Part model, mm, in its own coordinate system. Face numbers are marked on the shaded views. A direction names the side the tool comes from. Give positions to 0.01 mm unless a question says otherwise; leave off trailing zeros. Order: outer loops, then holes, each group sorted by start corner. A loop starts at its lowest first (then second) coordinate and runs counter-clockwise, first axis right, second up. Notation, with made-up numbers: M 26,33 L 31,33 A30 cw 31,58 Z; hole C 49.25,3.25 d8. An arc over 180 degrees is marked long. Return JSON: item names as keys, results as strings.
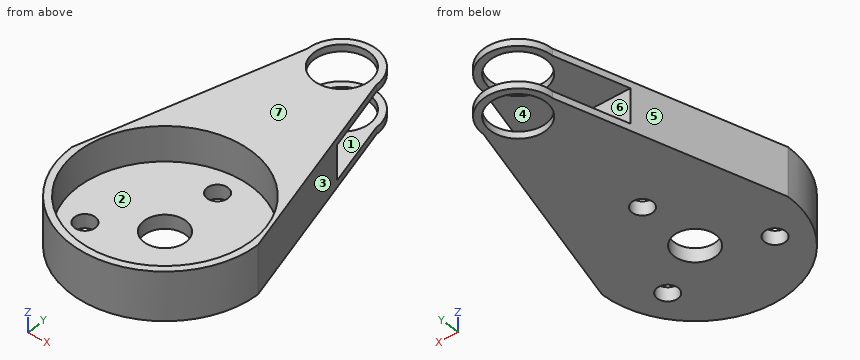
from build123d import *

# Parameters (mm, degrees)
BOSS_EXTRU_1_DEPTH      = 7
ESQUISSE2_R             = 3
ENL_V_MAT_EXTRU_1_DEPTH = 7
ESQUISSE3_R             = 1.5
ENL_V_MAT_EXTRU_2_DEPTH = 7
ESQUISSE4_R             = 4
ENL_V_MAT_EXTRU_3_DEPTH = 7
ESQUISSE5_R             = 12.5
ENL_V_MAT_EXTRU_4_DEPTH = 5
ESQUISSE6_W             = 27
ESQUISSE6_H             = 5
ENL_V_MAT_EXTRU_5_DEPTH = 20


with BuildPart() as part:
    # Esquisse1 → Boss.-Extru.1 (new body)
    with BuildSketch(Plane.XY):
        with BuildLine():
            Line((5, 0), (13.5, -30.265491901))
            ThreePointArc((13.5, -30.265491901), (0, -43.765491901), (-13.5, -30.265491901))
            Line((-13.5, -30.265491901), (-5, 0))
            ThreePointArc((-5, 0), (0, 5), (5, 0))
        make_face()
    extrude(amount=BOSS_EXTRU_1_DEPTH)

    # Esquisse2 → Enlèv. mat.-Extru.1 (cut)
    with BuildSketch(Plane.XY.offset(7)):
        with Locations((0, -30.265491901)):
            Circle(ESQUISSE2_R)
    extrude(amount=-ENL_V_MAT_EXTRU_1_DEPTH, mode=Mode.SUBTRACT)

    # Esquisse3 → Enlèv. mat.-Extru.2 (cut)
    with BuildSketch(Plane.XY.offset(7)):
        with Locations((0, -21.265491901)):
            Circle(ESQUISSE3_R)
        with Locations((-7.794228634, -34.765491901)):
            Circle(ESQUISSE3_R)
        with Locations((7.794228634, -34.765491901)):
            Circle(ESQUISSE3_R)
    extrude(amount=-ENL_V_MAT_EXTRU_2_DEPTH, mode=Mode.SUBTRACT)

    # Esquisse4 → Enlèv. mat.-Extru.3 (cut)
    with BuildSketch(Plane.XY.offset(7)):
        Circle(ESQUISSE4_R)
    extrude(amount=-ENL_V_MAT_EXTRU_3_DEPTH, mode=Mode.SUBTRACT)

    # Esquisse5 → Enlèv. mat.-Extru.4 (cut)
    with BuildSketch(Plane.XY.offset(7)):
        with Locations((0, -30.265491901)):
            Circle(ESQUISSE5_R)
    extrude(amount=-ENL_V_MAT_EXTRU_4_DEPTH, mode=Mode.SUBTRACT)

    # Esquisse6 → Enlèv. mat.-Extru.5 (cut)
    with BuildSketch(Plane(origin=(0, 10, 0), x_dir=(1, 0, 0), z_dir=(0, 1, 0))):
        with Locations((0, -3.5)):
            Rectangle(ESQUISSE6_W, ESQUISSE6_H)
    extrude(amount=-ENL_V_MAT_EXTRU_5_DEPTH, mode=Mode.SUBTRACT)


solid = part.part
Q1. Probe line 1 along Y through (x, z) = (0, 0.65); line 2 along Y through (x, z) = (0, 6.45); line 3 along Y through (x, z) = (0, 4.1). List the from-to ranges inside material, lowest first.
Established:
{"line 1": "y = -43.77 to -33.27, -27.27 to -22.77, -19.77 to -4, 4 to 5", "line 2": "y = -43.77 to -42.77, -17.77 to -4, 4 to 5", "line 3": "y = -43.77 to -42.77, -17.77 to -10"}
Q2. Band-saw the part on C-C (y = -32.5). Give the cut face in (x, z).
Established:
{"outline": "M -13.31,0 L -2,0 L -2,2 L -12.3,2 L -12.3,7 L -13.31,7 Z; M 2,0 L 13.31,0 L 13.31,7 L 12.3,7 L 12.3,2 L 2,2 Z"}
Q3. Band-saw the part on B-B (z = 3.5). Give the cut face in (x, y), then the cut area to 3 significant figures.
Established:
{"outline": "M -13.5,-30.27 A13.5 ccw 13.5,-30.27 L 7.81,-10 L -7.81,-10 Z; hole C 0,-30.27 d25", "area": "227 mm²"}
Q4. Band-saw the part on D-D (z = 6.5). Give the cut face in (x, y), then the cut area to 3 significant figures.
Established:
{"outline": "M -13.5,-30.27 A13.5 ccw 13.5,-30.27 L 5,0 A5 ccw -5,0 Z; hole C 0,-30.27 d25; hole C 0,0 d8", "area": "344 mm²"}
Q5. 3-axis set-ups, long thin cutter, end or side, ignore diameter. For the marked faces 1, 2 and 3: which of +Z, -Z, +X, -X, +Y, -Y reach the whole face in a straight line?
Established:
{"face 1": "+X, -X, +Y", "face 2": "+Z", "face 3": "+Z, -Z, +X, +Y"}
Q6. Pin check, flat tips, straight feed: pin 1 (2 mm diameter, centred on x = 3, z = 1.5, fed in from -Y); pin 2 (2.5 mm diameter, centred on x = -7.79, y = -34.77, fed in from -Z); pin 3 (1 mm diameter, centred on x = 3.5, z = 2.5, fed in from +Y); pin 4 (10.5 mm diameter, centred on x = 0, y = 0, fed in from +Z). Stop position of each tip, or through.
Established:
{"pin 1": "stops at y = -43.62", "pin 2": "passes through", "pin 3": "stops at y = -10", "pin 4": "stops at z = 7"}
Q7. Two-plate mould, pull along Z, no slides. Class the marked faces 4, 5, 6 and 7: +Z half, -Z half, draft (parallel to the pull), parting line (faces both ways), or undercut.
Established:
{"face 4": "undercut", "face 5": "draft", "face 6": "undercut", "face 7": "+Z half"}
Q8. Band-saw the part on A-A (x = 0). Give the cut face in (y, z), then the cut area to 3 significant figures.
Established:
{"outline": "M -43.77,0 L -33.27,0 L -33.27,2 L -42.77,2 L -42.77,7 L -43.77,7 Z; M -27.27,0 L -22.77,0 L -22.77,2 L -27.27,2 Z; M -19.77,0 L -4,0 L -4,1 L -10,1 L -10,6 L -4,6 L -4,7 L -17.77,7 L -17.77,2 L -19.77,2 Z; M 4,0 L 5,0 L 5,1 L 4,1 Z; M 4,6 L 5,6 L 5,7 L 4,7 Z", "area": "107 mm²"}
